Answer from the drawing. Dimensions are ordinates in mm from the lowest x, y and z of the part. A direction names the side the tool comes from. Give positions to 0.01 mm unless a question says otherwise; leave off trailing zeros. Order: outer loops, then holes, each group sorted by start corner. A loop starts at its lowest first (then second) coordinate and runs counter-clockwise, first axis right, second up. Notation, with made-up numbers: (-29.5, -38) - (-2.5, -38) arc R12 cw to (-2.5, -31) - close; hole circle Ø1 at (19, 23). An arc over 180 degrees is marked (long way). Use a Markdown table: item, result. Add a question column.
1) Find section A-A, the plane x = 125. Determine the outline of the cut face in (y, z), plus the area to 3 significant figures.
2) Flat-ended cylindrical pins translate along their axes: pin 1 (3 mm diameter, centred on y = 142.5, z = 10.5, fed in from +X); pin 2 (12 mm diameter, centred on x = 170, y = 77.5, fed in from +Z); pin 3 (8 mm diameter, centred on y = 167.5, z = 16, fed in from +X). Find the tip coordinate at first contact, or state that the pin passes through.
3) For the marked faces 1 and 2, determine the directions among +Z, -Z, +X, -X, +Y, -Y from which every point of the face is accessible in a straight line to the end or side of a thin tool.
4) Find section C-C, the plane z = 41.5. Determine the outline of the cut face in (x, y), plus the area to 3 significant figures.
5) Straight lines are drawn through the part: line 1 (Z direction, x = 41, y = 110.5); line 2 (Z direction, x = 11.5, y = 171); line 3 (Y direction, x = 146.5, z = 35). For each, find the intervals that lie inside material, in ascending order.
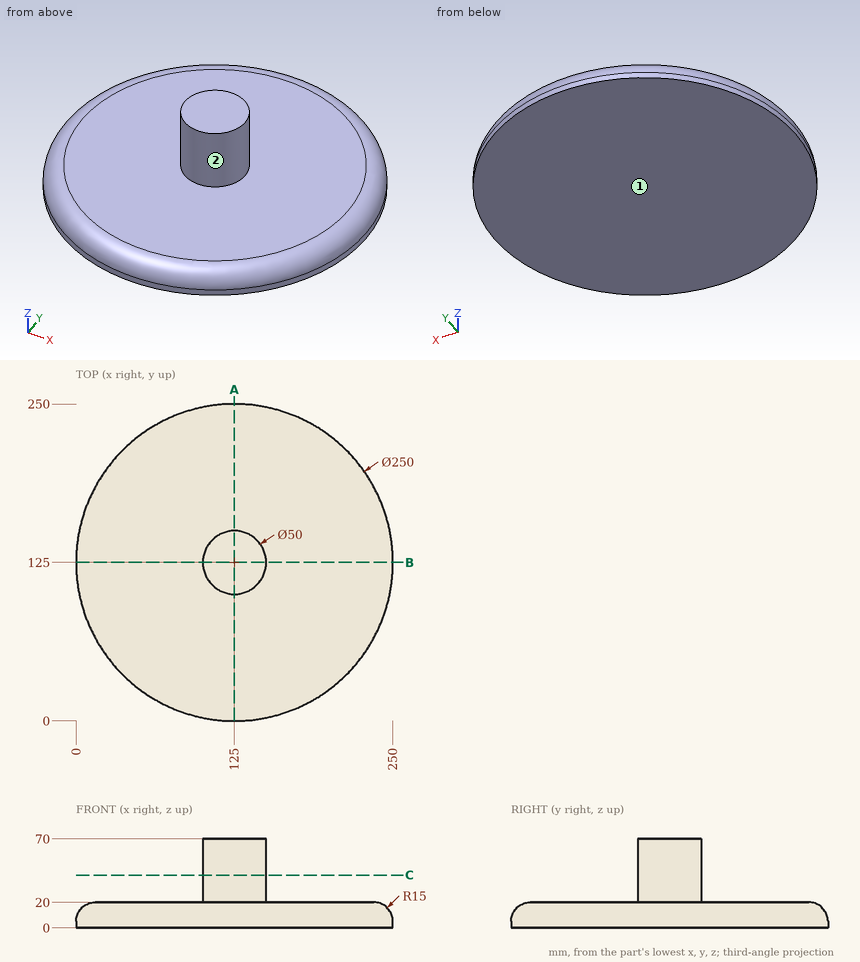
The answers:
| question | item | result |
|---|---|---|
| 1 | outline | (0, 0) - (250, 0) - (250, 5) arc R15 ccw to (235, 20) - (150, 20) - (150, 70) - (100, 70) - (100, 20) - (15, 20) arc R15 ccw to (0, 5) - close |
| 1 | area | 7,400 mm2 |
| 2 | pin 1 | x = 248.27 |
| 2 | pin 2 | z = 20 |
| 2 | pin 3 | x = 241.11 |
| 3 | face 1 | -Z, +X, -X, +Y, -Y |
| 3 | face 2 | +Z |
| 4 | outline | circle Ø50 at (125, 125) |
| 4 | area | 1,960 mm2 |
| 5 | line 1 | 0 to 20 |
| 5 | line 2 | 0 to 13.34 |
| 5 | line 3 | 112.24 to 137.76 |
